Autodesk Inventor part; units mm, degrees
ref_plane "YZ Plane" through (0, 0, 0) normal (1, 0, 0) x (0, 1, 0)
ref_plane "XZ Plane" through (0, 0, 0) normal (0, 1, 0) x (-1, 0, 0)
ref_plane "XY Plane" through (0, 0, 0) normal (0, 0, 1) x (1, 0, 0)
sketch "Sketch1" plane through (0, 0, 0) normal (0, 1, 0) x (-1, 0, 0)
  line L0 (5, 14.75) -> (-5, 14.75)
  line L1 (-5, 14.75) -> (-5, -14.75)
  line L2 (-5, -14.75) -> (5, -14.75)
  line L3 (5, -14.75) -> (5, 14.75)
  line L4 (5, 14.75) -> (-5, -14.75) construction
  line L5 (-5, 14.75) -> (5, -14.75) construction
  point P0 (0, 0)
  dimension "d0" = 10
  dimension "d1" = 29.5
extrude "Extrusion1" add sketch "Sketch1" along normal blind 2
sketch "Sketch2" plane through (0, 2, 0) normal (0, 1, 0) x (1, 0, 0)
  line L0 (5, 14.75) -> (-5, 14.75)
  line L1 (5, -14.75) -> (5, 14.75)
  line L2 (-5, 14.75) -> (5, 14.75)
  line L3 (5, 14.75) -> (5, 12.75)
  line L4 (5, 12.75) -> (-5, 12.75)
  line L5 (-5, 12.75) -> (-5, 14.75)
  point P0 (0, 0)
  dimension "d4" = 2
extrude "Extrusion2" add sketch "Sketch2" along normal blind 15
sketch "Sketch3" plane through (-5, 2, -12.75) normal (0, 0, 1) x (1, 0, 0)
  circle A0 centre (5, 12) radius 1.5
  circle A1 centre (5, 2) radius 1.5
  line L0 (0, 0) -> (10, 0)
  point P0 (5, -2)
  dimension "d7" = 3
  dimension "d8" = 3
  dimension "d9" = 2
  dimension "d10" = 10
extrude "Extrusion3" cut sketch "Sketch3" against normal blind 15
properties part number "Bracket Lifter Motor 2"
Verification items for the finished model (mm, model axes). A direction names the side the tool comes from. Give positions to 0.01 mm unless a question says otherwise; leave off trailing zeros. Loops run counter-clockwise (first coordinate to the right, second up) from the corner with the lowest first, then second, coordinate; pieces in that order, holes last.
1. Section check C-C, the plane z = 3. Enter the section's corners in (x, y).
2. Thickness scan on line 1 (Y direction, x = 0, z = -13.9); line 2 (Y direction, x = -3.25, z = -5.5); line 3 (Z direction, x = 4, y = 12.5). Record the ranges inside material, lowest first.
3. Section check D-D, the plane y = 6.25. Enter the section's corners in (x, z).
4. Mould release check, pull along Y, two halves, no side actions. Record for faces 1 (the flat face through (0, 17, -14)), 2 (the cylindrical face through (0.806, 5.265, -13.736)), 3 (the flat face through (5, 1.5, -5.4)): released by +Y, released by -Y, zero draft, split by the parting line, or undercut.
5. Section check B-B, the plane y = 4. Enter the section's corners in (x, z).
6. Set-up check for faces 4 (the flat face through (0, 8, -14.75)), 5 (the flat face through (0, 2, 1)): record each of +Z, -Z, +X, -X, +Y, -Y from which the full face is reachable in a straight line by a thin tool's end or side.
7. Go/stop test with flat-tipped pins: pin 1 Ø4 at (x, y) = (-3, 10.5) entering from +Z; pin 2 Ø3 at (x, z) = (0.5, -9) entering from +Y. Record where each tip stops, or that it passes through.
8. Section check A-A, the plane x = 0. Enter the section's corners in (y, z).
Geometry says:
1. outline: (-5, 0) - (5, 0) - (5, 2) - (-5, 2) - close
2. line 1: y = 0 to 2.5, 5.5 to 12.5, 15.5 to 17
2. line 2: y = 0 to 2
2. line 3: z = -14.75 to -12.75
3. outline: (-5, -14.75) - (5, -14.75) - (5, -12.75) - (-5, -12.75) - close
4. face 1: released by +Y
4. face 2: undercut
4. face 3: zero draft
5. outline: (-5, -14.75) - (-1.5, -14.75) - (-1.5, -12.75) - (-5, -12.75) - close; (1.5, -14.75) - (5, -14.75) - (5, -12.75) - (1.5, -12.75) - close
6. face 4: -Z, +X, -X, +Y, -Y
6. face 5: +Z, +X, -X, +Y
7. pin 1: stops at z = -12.75
7. pin 2: stops at y = 2
8. outline: (0, -14.75) - (2.5, -14.75) - (2.5, -12.75) - (2, -12.75) - (2, 14.75) - (0, 14.75) - close; (5.5, -14.75) - (12.5, -14.75) - (12.5, -12.75) - (5.5, -12.75) - close; (15.5, -14.75) - (17, -14.75) - (17, -12.75) - (15.5, -12.75) - close
